Autodesk Inventor part; units mm, degrees
ref_plane "YZ Plane" through (0, 0, 0) normal (1, 0, 0) x (0, 1, 0)
ref_plane "XZ Plane" through (0, 0, 0) normal (0, 1, 0) x (-1, 0, 0)
ref_plane "XY Plane" through (0, 0, 0) normal (0, 0, 1) x (1, 0, 0)
sketch "Sketch1" plane through (0, 0, 0) normal (0, 0, 1) x (1, 0, 0)
  line L0 (-25.35, -16.9) -> (25.35, -16.9)
  line L1 (25.35, -16.9) -> (25.35, 16.9)
  line L2 (25.35, 16.9) -> (-25.35, 16.9)
  line L3 (-25.35, 16.9) -> (-25.35, -16.9)
  line L4 (-25.35, -16.9) -> (25.35, 16.9) construction
  line L5 (25.35, -16.9) -> (-25.35, 16.9) construction
  point P0 (0, 0)
  dimension "d0" = 50.7
  dimension "d1" = 33.8
extrude "Extrusion1" add sketch "Sketch1" along normal blind 42.5
sketch "Sketch3" plane through (0, 0, 0) normal (1, 0, 0) x (0, 1, 0)
  line L0 (16.9, 42.5) -> (16.9, 0)
  line L1 (16.9, 0) -> (-16.9, 0)
  line L2 (-16.9, 0) -> (-16.9, 42.5)
  line L3 (-16.9, 42.5) -> (16.9, 42.5)
  line L4 (16.9, 42.5) -> (16.9, 43.5)
  line L5 (16.9, 43.5) -> (-17.1, 43.5)
  line L6 (-17.1, 43.5) -> (-17.1, 54)
  line L7 (-17.1, 54) -> (-18.1, 54)
  line L8 (-18.1, 54) -> (-18.1, 43.5)
  line L9 (-17.1, 42.5) -> (-16.9, 42.5)
  arc A0 (-18.1, 43.5) -> (-17.1, 42.5) centre (-17.1, 43.5) ccw
  point P0 (0, 0)
  dimension "d4" = 1
  dimension "d5" = 1
  dimension "d6" = 35
  dimension "d7" = 1
  dimension "d8" = 54
extrude "Extrusion2" add sketch "Sketch3" along normal mid plane 35 contours L3 L9 A0 L8 L7 L6 L5 L4
fillet "Fillet2" radius 2.5 4 edges at (25.35, -16.9, 21.25) (25.35, 16.9, 21.25) (-25.35, 16.9, 21.25) (-25.35, -16.9, 21.25)
sketch "Sketch4" plane through (-17.5, -17.1, 54) normal (0, 1, 0) x (1, 0, 0)
  line L0 (17.5, 54) -> (17.5, 4) construction
  line L1 (4, 4) -> (31, 4) construction
  circle A0 centre (4, 4) radius 2
  circle A1 centre (31, 4) radius 2
  dimension "d13" = 4
  dimension "d14" = 50
  dimension "d15" = 27
extrude "Extrusion3" cut sketch "Sketch4" against normal through all
mirror "Mirror1" about plane through (0, 0, 0) normal (0, 0, 1)
properties part number "esc"
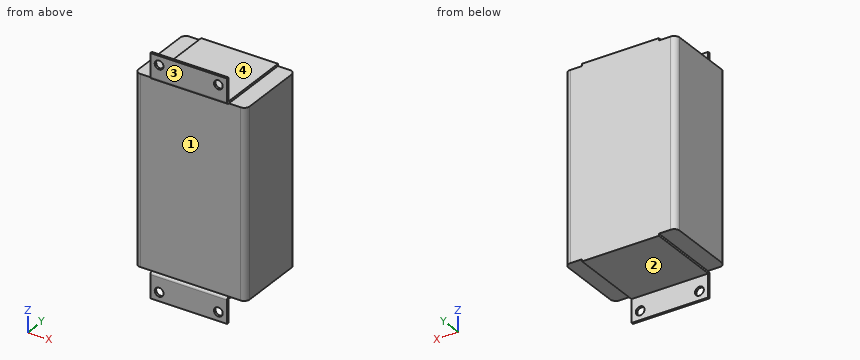
Work out the finished part from the listing and answer in its coordinate system (mm). Face numbers are marked on the shaded views. A direction names the side the tool comes from. Round coordinates to 2 decimals unless told otherwise and drop trailing zeros. Write each loop counter-clockwise with the first axis right and the second up, starting at its lowest first coordinate (ties: lowest second). Pieces come first, ordered by that corner, then holes.
1) A cutting plane is placed at D-D (x = 2). Give the vertices of the cut face in (y, z), plus the area to 3 significant figures.
2) A cutting plane is placed at C-C (z = -17). Give the vertices of the cut face in (x, y), plus the area to 3 significant figures.
3) Straight lines are drawn through the part: line 1 (X direction, y = -17.75, z = 50); line 2 (Y direction, x = -4.5, z = 47); line 3 (Z direction, x = 21.5, y = -1). For each, find the intervals that lie inside material, in ascending order.
4) A cutting plane is placed at A-A (x = -13.5). Give the vertices of the cut face in (y, z), plus the area to 3 significant figures.
5) A tool of negligible diameter and unlimited length cuts with its end or side. For the marked faces 1, 2, 3 and 4, from which of +Z, -Z, +X, -X, +Y, -Y can it reach the whole face along a straight path? Write none if from no direction.
6) A cutting plane is placed at B-B (z = -50). Give the vertices of the cut face in (x, y), plus the area to 3 significant figures.
7) Given pin 1 Ø4 at (x, z) = (-13.5, -9) entering from -Y; pin 2 Ø8.5 at (x, y) = (-22.5, 8) entering from +Z; pin 3 Ø5 at (x, y) = (-13, 0.5) entering from -Z; pin 4 Ø11.5 at (x, z) = (-2.5, -47.5) entering from +Y, each flat-ended and moving along its own axis, determine where each tip first touches the part or whether it passes through.
Completed:
1. outline: (-18.1, -54) - (-17.1, -54) - (-17.1, -43.5) - (16.9, -43.5) - (16.9, 43.5) - (-17.1, 43.5) - (-17.1, 54) - (-18.1, 54) - (-18.1, 43.5) arc R1 ccw to (-17.1, 42.5) - (-16.9, 42.5) - (-16.9, -42.5) - (-17.1, -42.5) arc R1 ccw to (-18.1, -43.5) - close
1. area: 2,960 mm2
2. outline: (-25.35, -14.4) arc R2.5 ccw to (-22.85, -16.9) - (22.85, -16.9) arc R2.5 ccw to (25.35, -14.4) - (25.35, 14.4) arc R2.5 ccw to (22.85, 16.9) - (-22.85, 16.9) arc R2.5 ccw to (-25.35, 14.4) - close
2. area: 1,710 mm2
3. line 1: x = -17.5 to -15.5, -11.5 to 11.5, 15.5 to 17.5
3. line 2: y = -18.1 to -17.1
3. line 3: z = -42.5 to 42.5
4. outline: (-18.1, -54) - (-17.1, -54) - (-17.1, -52) - (-18.1, -52) - close; (-18.1, -48) - (-17.1, -48) - (-17.1, -43.5) - (16.9, -43.5) - (16.9, 43.5) - (-17.1, 43.5) - (-17.1, 48) - (-18.1, 48) - (-18.1, 43.5) arc R1 ccw to (-17.1, 42.5) - (-16.9, 42.5) - (-16.9, -42.5) - (-17.1, -42.5) arc R1 ccw to (-18.1, -43.5) - close; (-18.1, 52) - (-17.1, 52) - (-17.1, 54) - (-18.1, 54) - close
4. area: 2,960 mm2
5. face 1: +X, -X, -Y
5. face 2: -Z, +X, -X, +Y
5. face 3: +Z, -Z, +X, -X, -Y
5. face 4: +Z, +X, -X, +Y
6. outline: (-17.5, -18.1) - (-15.5, -18.1) - (-15.5, -17.1) - (-17.5, -17.1) - close; (-11.5, -18.1) - (11.5, -18.1) - (11.5, -17.1) - (-11.5, -17.1) - close; (15.5, -18.1) - (17.5, -18.1) - (17.5, -17.1) - (15.5, -17.1) - close
6. area: 27.0 mm2
7. pin 1: stops at y = -16.9
7. pin 2: stops at z = 42.5
7. pin 3: stops at z = -43.5
7. pin 4: stops at y = 16.9
